Work out the finished part from the listing and answer in its coordinate system (mm). Coordinates: 2 decimals unless noted, no trailing zeros. Order: outer loops, then holes, each group sorted by start corner. A loop starts at its lowest first (then second) coordinate and runs counter-clockwise, first axis right, second up. Notation, with made-up numbers: M 74.25,-6 L 102.25,-6 A25 ccw 102.25,22 Z; hole C 70,26.25 d1. An arc over 180 degrees is marked long. Use a Markdown table: item, result.
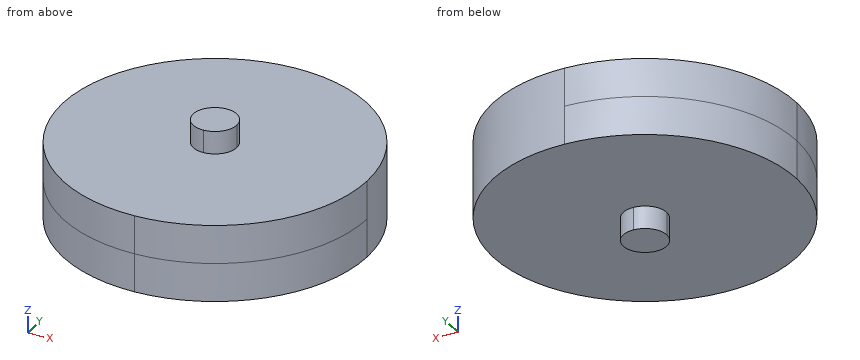
from build123d import *

# Parameters (mm, degrees)
F1_DEPTH = 2.2
F2_DEPTH = 3.5


with BuildPart() as f1:
    # F0 (on Top) → F1 (new body, symmetric)
    with BuildSketch(Plane.XY):
        with BuildLine():
            Line((-27.9816011338, 0), (-20.5316011338, 0))
            ThreePointArc((-20.5316011338, 0), (-23.0797721375, 6.1518289963), (-29.2316011338, 8.7))
            Line((-29.2316011338, 8.7), (-29.2316011338, 1.25))
            ThreePointArc((-29.2316011338, 1.25), (-28.3477176573, 0.8838834765), (-27.9816011338, 0))
        make_face()
        with BuildLine():
            Line((-29.2316011338, 1.25), (-29.2316011338, 8.7))
            ThreePointArc((-29.2316011338, 8.7), (-35.3834301302, 6.1518289963), (-37.9316011338, 0))
            Line((-37.9316011338, 0), (-30.4816011338, 0))
            ThreePointArc((-30.4816011338, 0), (-30.1154846103, 0.8838834765), (-29.2316011338, 1.25))
        make_face()
        with BuildLine():
            ThreePointArc((-37.9316011338, 0), (-35.3834301302, -6.1518289963), (-29.2316011338, -8.7))
            Line((-29.2316011338, -8.7), (-29.2316011338, -1.25))
            ThreePointArc((-29.2316011338, -1.25), (-30.1154846103, -0.8838834765), (-30.4816011338, 0))
            Line((-30.4816011338, 0), (-37.9316011338, 0))
        make_face()
        with BuildLine():
            ThreePointArc((-29.2316011338, -8.7), (-23.0797721375, -6.1518289963), (-20.5316011338, 0))
            Line((-20.5316011338, 0), (-27.9816011338, 0))
            ThreePointArc((-27.9816011338, 0), (-28.3477176573, -0.8838834765), (-29.2316011338, -1.25))
            Line((-29.2316011338, -1.25), (-29.2316011338, -8.7))
        make_face()
    extrude(amount=F1_DEPTH, both=True)

    # F0 (on Top) → F2 (join, symmetric)
    with BuildSketch(Plane.XY):
        with BuildLine():
            ThreePointArc((-29.2316011338, -1.25), (-28.3477176573, -0.8838834765), (-27.9816011338, 0))
            Line((-27.9816011338, 0), (-29.2316011338, 0))
            Line((-29.2316011338, 0), (-29.2316011338, -1.25))
        make_face()
        with BuildLine():
            Line((-29.2316011338, 0), (-27.9816011338, 0))
            ThreePointArc((-27.9816011338, 0), (-28.3477176573, 0.8838834765), (-29.2316011338, 1.25))
            Line((-29.2316011338, 1.25), (-29.2316011338, 0))
        make_face()
        with BuildLine():
            Line((-29.2316011338, 0), (-29.2316011338, 1.25))
            ThreePointArc((-29.2316011338, 1.25), (-30.1154846103, 0.8838834765), (-30.4816011338, 0))
            Line((-30.4816011338, 0), (-29.2316011338, 0))
        make_face()
        with BuildLine():
            ThreePointArc((-30.4816011338, 0), (-30.1154846103, -0.8838834765), (-29.2316011338, -1.25))
            Line((-29.2316011338, -1.25), (-29.2316011338, 0))
            Line((-29.2316011338, 0), (-30.4816011338, 0))
        make_face()
    extrude(amount=F2_DEPTH, both=True)


solid = f1.part
1. Find the intervals of material crossed by probe 1 along Z at (x, y) = (-30.5, 1); probe 2 along X at (y, z) = (-7, -1.75); probe 3 along Y at (x, z) = (-23.5, 0.5), in increasing order.
Answers below:
| item | result |
|---|---|
| probe 1 | -2.2 to 2.2 |
| probe 2 | -34.4 to -24.07 |
| probe 3 | -6.55 to 6.55 |
2. Flat-ended cylindrical pins translate along their axes: P1, Ø2, axis at y = -6, z = -1, coming from the +X side; P2, Ø1, axis at x = -32.5, z = 0.5, coming from the +Y side; P3, Ø2, axis at y = 6.5, z = 0.5, coming from the +X side. Find the tip coordinate at first contact, or state that the pin passes through.
Answers below:
| item | result |
|---|---|
| P1 | x = -22.11 |
| P2 | y = 8.25 |
| P3 | x = -22.49 |
3. Section C-C on y = 5 is taken. Determine the outline of the cut face in (x, z).
Answers below:
| item | result |
|---|---|
| outline | M -36.35,-2.2 L -22.11,-2.2 L -22.11,2.2 L -36.35,2.2 Z |
4. Section B-B on z = 0.5 is taken. Determine the outline of the cut face in (x, y).
Answers below:
| item | result |
|---|---|
| outline | C -29.23,0 d17.4 |
5. Section D-D on x = -30 is taken. Determine the outline of the cut face in (y, z).
Answers below:
| item | result |
|---|---|
| outline | M -8.67,-2.2 L -0.99,-2.2 L -0.99,-3.5 L 0.99,-3.5 L 0.99,-2.2 L 8.67,-2.2 L 8.67,2.2 L 0.99,2.2 L 0.99,3.5 L -0.99,3.5 L -0.99,2.2 L -8.67,2.2 Z |
6. Section A-A on x = -28.25 is taken. Determine the outline of the cut face in (y, z), then the cut area to 3 significant figures.
Answers below:
| item | result |
|---|---|
| outline | M -8.64,-2.2 L -0.77,-2.2 L -0.77,-3.5 L 0.77,-3.5 L 0.77,-2.2 L 8.64,-2.2 L 8.64,2.2 L 0.77,2.2 L 0.77,3.5 L -0.77,3.5 L -0.77,2.2 L -8.64,2.2 Z |
| area | 80.1 mm² |
